Source: CAD feature listing. Evaluate the final solid. Frame: model axes, mm. A direction names the side the tool comes from. Give positions to 0.01 mm unless a question says otherwise; leave off trailing zeros. Order: outer loops, then holes, each group sorted by start corner. A loop starts at its lowest first (then second) coordinate and runs counter-clockwise, first axis right, second up. Notation, with made-up numbers: (51, 32) -> (71, 32) arc R26 cw to (71, 63) -> close; hole circle Ø6 at (-26, 11). An arc over 180 degrees is marked (long way). Answer in a Markdown table with one row per item.
Autodesk Inventor part; units mm, degrees
ref_plane "YZ Plane" through (0, 0, 0) normal (1, 0, 0) x (0, 1, 0)
ref_plane "XZ Plane" through (0, 0, 0) normal (0, 1, 0) x (-1, 0, 0)
ref_plane "XY Plane" through (0, 0, 0) normal (0, 0, 1) x (1, 0, 0)
sketch "Sketch1" plane through (0, 0, 0) normal (0, 1, 0) x (-1, 0, 0)
  line L0 (21.5, -10.6) -> (-21.5, -10.6)
  line L1 (-21.5, -10.6) -> (-21.5, 10.6)
  line L2 (-21.5, 10.6) -> (21.5, 10.6)
  line L3 (21.5, 10.6) -> (21.5, -10.6)
  point P0 (0, 0)
  dimension "d0" = 43
  dimension "d1" = 21.2
  dimension "d2" = 10.6
  dimension "d3" = 21.5
extrude "Extrusion1" add sketch "Sketch1" along normal blind 1.31
sketch "Sketch2" plane through (0, 1.31, 0) normal (0, 1, 0) x (1, 0, 0)
  line L0 (-12, 10) -> (-1.85, 10)
  line L1 (-1.85, 10) -> (-1.85, -2.4)
  line L2 (-1.85, -2.4) -> (-12, -2.4)
  line L3 (-12, -2.4) -> (-12, 10)
  line L4 (-21.5, -10.6) -> (21.5, -10.6)
  line L5 (-21.5, 10.6) -> (-21.5, -10.6)
  point P0 (0, 0)
  dimension "d6" = 12.4
  dimension "d7" = 10.15
  dimension "d8" = 8.2
  dimension "d9" = 9.5
extrude "Extrusion2" add sketch "Sketch2" along normal blind 4
sketch "Sketch3" plane through (0, 1.31, 0) normal (0, 1, 0) x (1, 0, 0)
  line L0 (0.6, 2.8) -> (10.8, 2.8)
  line L1 (11.8, 1.8) -> (11.8, -8.4)
  line L2 (10.8, -9.4) -> (0.6, -9.4)
  line L3 (-0.4, -8.4) -> (-0.4, 1.8)
  line L4 (-21.5, -10.6) -> (21.5, -10.6)
  line L5 (21.5, -10.6) -> (21.5, 10.6)
  arc A0 (0.6, 2.8) -> (-0.4, 1.8) centre (0.6, 1.8) ccw
  arc A1 (11.8, 1.8) -> (10.8, 2.8) centre (10.8, 1.8) ccw
  arc A2 (10.8, -9.4) -> (11.8, -8.4) centre (10.8, -8.4) ccw
  arc A3 (-0.4, -8.4) -> (0.6, -9.4) centre (0.6, -8.4) ccw
  point P0 (0, 0)
  dimension "d12" = 12.2
  dimension "d13" = 12.2
  dimension "d14" = 1.2
  dimension "d15" = 9.7
  dimension "d16" = 1
extrude "Extrusion3" add sketch "Sketch3" along normal blind 7.4
sketch "Sketch4" plane through (0, 1.31, 0) normal (0, 1, 0) x (1, 0, 0)
  line L0 (2.66, 10.1) -> (12.13, 10.1)
  line L1 (12.13, 10.1) -> (12.13, 5.79)
  line L2 (12.13, 5.79) -> (2.66, 5.79)
  line L3 (2.66, 5.79) -> (2.66, 10.1)
  line L4 (21.5, -10.6) -> (21.5, 10.6)
  line L5 (21.5, 10.6) -> (-21.5, 10.6)
  point P0 (0, 0)
  dimension "d19" = 4.31
  dimension "d20" = 9.47
  dimension "d21" = 9.37
  dimension "d22" = 0.5
extrude "Extrusion4" add sketch "Sketch4" along normal blind 10
sketch "Sketch5" plane through (0, 11.31, 0) normal (0, 1, 0) x (1, 0, 0)
  circle A0 centre (3.86, 8.9) radius 1.125
  line L0 (12.13, 10.1) -> (2.66, 10.1)
  line L1 (2.66, 10.1) -> (2.66, 5.79)
  point P0 (0, 0)
  point P1 (2.66, 9.2358)
  point P2 (2.66, 8.7642)
  point P3 (4.0958, 10.1)
  point P4 (3.6242, 10.1)
  dimension "d25" = 2.25
  dimension "d26" = 1.2
  dimension "d27" = 1.2
extrude "Extrusion5" add sketch "Sketch5" along normal blind 1.61
sketch "Sketch6" plane through (0, 1.31, 0) normal (0, 1, 0) x (1, 0, 0)
  circle A0 centre (-16.28, 0.87) radius 4
  circle A1 centre (16.93, 1.23) radius 4
  line L0 (-21.5, -10.6) -> (21.5, -10.6)
  line L1 (21.5, -10.6) -> (21.5, 10.6)
  line L2 (-21.5, 10.6) -> (-21.5, -10.6)
  point P0 (0, 0)
  dimension "d30" = 8
  dimension "d31" = 8
  dimension "d32" = 11.83
  dimension "d33" = 4.57
  dimension "d34" = 5.22
  dimension "d35" = 11.47
extrude "Extrusion6" add sketch "Sketch6" along normal blind 10.5
fillet "Fillet1" radius 0.5 2 edges at (12.93, 11.81, -1.23) (-20.28, 11.81, -0.87)
properties part number "Control and Power Box"
(1) Section query A-A (y = 10.75). Return the cut outline in (x, z).
A:
| item | result |
|---|---|
| outline | circle Ø8 at (-16.28, -0.87); (2.66, -10.1) -> (12.13, -10.1) -> (12.13, -5.79) -> (2.66, -5.79) -> close; circle Ø8 at (16.93, -1.23) |
(2) Ray query, probe 1 along X at (y, z) = (8.5, -1); probe 2 along X at (y, z) = (2.75, 2); probe 3 along X at (y, z) = (2.75, 0.75). Return the intervals inside material, ascending.
A:
| item | result |
|---|---|
| probe 1 | x = -20.28 to -12.28, -0.4 to 11.8, 12.94 to 20.92 |
| probe 2 | x = -19.07 to -13.49, -12 to -1.85, -0.4 to 11.8, 14.57 to 19.29 |
| probe 3 | x = -19.94 to -12.62, -12 to -1.85, -0.4 to 11.8, 13.45 to 20.41 |
(3) Access query for faces 4 (the flat face through (-7, 3, -10)), 5 (the flat face through (7, 6, -5.79)), 6 (the cylindrical face through (11.499, 4.958, -2.515)). Directions: +Z, -Z, +X, -X, +Y, -Y. A direction counts if a zero-diameter tool reaches every point of the face in a straight line with its end or side. Return the directions, or none.
A:
| item | result |
|---|---|
| face 4 | -Z, -X, +Y |
| face 5 | +X, +Y |
| face 6 | +Y |
(4) Section query C-C (x = -10). Return the cut outline in (y, z), plus the area to 3 significant figures.
A:
| item | result |
|---|---|
| outline | (0, -10.6) -> (1.31, -10.6) -> (1.31, -10) -> (5.31, -10) -> (5.31, 2.4) -> (1.31, 2.4) -> (1.31, 10.6) -> (0, 10.6) -> close |
| area | 77.4 mm^2 |
(5) First-contact query: pin 1 Ø6 at (x, y) = (-5, 8) entering from -Z; pin 2 Ø12 at (x, z) = (3.5, 4) entering from +Y; pin 3 Ø2 at (x, z) = (16.5, -3) entering from +Y. Flat tips, straight axial feed; report the tip coordinate or a pass-through.
A:
| item | result |
|---|---|
| pin 1 | stops at z = -10 |
| pin 2 | stops at y = 8.71 |
| pin 3 | stops at y = 11.81 |
(6) Section query D-D (z = 5.5). Return the cut outline in (x, y).
A:
| item | result |
|---|---|
| outline | (-21.5, 0) -> (21.5, 0) -> (21.5, 1.31) -> (11.8, 1.31) -> (11.8, 8.71) -> (-0.4, 8.71) -> (-0.4, 1.31) -> (-21.5, 1.31) -> close |
(7) Section query B-B (y = 8). Return the cut outline in (x, z).
A:
| item | result |
|---|---|
| outline | circle Ø8 at (-16.28, -0.87); (-0.4, -1.8) arc R1 ccw to (0.6, -2.8) -> (10.8, -2.8) arc R1 ccw to (11.8, -1.8) -> (11.8, 8.4) arc R1 ccw to (10.8, 9.4) -> (0.6, 9.4) arc R1 ccw to (-0.4, 8.4) -> close; (2.66, -10.1) -> (12.13, -10.1) -> (12.13, -5.79) -> (2.66, -5.79) -> close; circle Ø8 at (16.93, -1.23) |
(8) Pull-direction query (X, two-part tool) for faces 1 (the flat face through (0, 0, 0)), 2 (the flat face through (2.66, 6, -8)), 3 (the flat face through (-21.5, 1, 0)); classes: +X half, -X half, draft (parallel to the pull), parting line (faces both ways), or undercut.
A:
| item | result |
|---|---|
| face 1 | draft |
| face 2 | undercut |
| face 3 | -X half |
